The model under review builds one solid part; all positions refer to its coordinate system, in mm. A direction names the side the tool comes from. Coordinates: 2 decimals unless noted, no trailing zeros. Order: outer loops, then holes, each group sorted by start corner. A loop starts at its lowest first (then second) coordinate and runs counter-clockwise, first axis right, second up. Notation, with made-up numbers: M -24,62 L -17,62 A18 ccw -17,81 Z; hole C -6.75,75 d6. An arc over 180 degrees is marked long. One line per item, written item: value.
```python
from build123d import *

# Parameters (mm, degrees)
FILLET1_R          = 0.2
SKETCH2_W          = 1
SKETCH2_H          = 6.101946446
CUT_EXTRUDE1_DEPTH = 1


with BuildPart() as part:
    # Sketch1 → Revolve1 (revolve)
    with BuildSketch(Plane.XY, mode=Mode.PRIVATE) as revolve1_sk:
        Polygon((-6.402554748, 1.5), (-43, 1.5), (-43, 0), (16, 0), (20, 0), (20, 2.75), (18.5, 2.75), (18.5, 1.25), (16, 1.25), (16, 4), (0, 4), (0, 3.603313767), (-1.581765583, 2.560980975), align=None)
    revolve(revolve1_sk.sketch.rotate(Axis((-43, 0, 0), (1, 0, 0)), 90), axis=Axis((-43, 0, 0), (1, 0, 0)))

    # Fillet1
    fillet1_edges = [part.edges().sort_by_distance(p)[0] for p in [
        (0, 0, -4),
        (16, 0, -4),
    ]]
    fillet(fillet1_edges, radius=FILLET1_R)

    # Sketch2 → Cut-Extrude1 (cut)
    with BuildSketch(Plane(origin=(20, 0, 0), x_dir=(0, 0, -1), z_dir=(1, 0, 0))):
        with Locations((0, 0.058366444)):
            Rectangle(SKETCH2_W, SKETCH2_H)
    extrude(amount=-CUT_EXTRUDE1_DEPTH, mode=Mode.SUBTRACT)


solid = part.part
```
(1) Tool access review of faces 4 (the flat face through (16, -1, 1)), 5 (the cylindrical face through (-24.96, -0.45, 1.43)), 6 (the cylindrical face through (19.24, 2.44, 1.27)), 7 (the flat face through (19.5, 0, 0.5)), 8 (the flat face through (20, 0, -1)): name each direction out of +Z, -Z, +X, -X, +Y, -Y from which nothing blocks a thin tool from reaching the whole face with its end or side.
Geometry results:
face 4: none
face 5: -X
face 6: +X
face 7: +X, +Y, -Y
face 8: +Z, -Z, +X, +Y, -Y
(2) Mouldability with a two-part tool opening along X and no side actions: class faces 1 (the flat face through (19.5, 0, -0.5)), 2 (the conical face through (-4.6, -0.6, 1.8)), 3 (the cylindrical face through (17.23, -0.05, -1.25)) as +X half, -X half, draft (parallel to the pull), parting line (faces both ways), or undercut.
Geometry results:
face 1: draft
face 2: -X half
face 3: undercut
(3) We need section A-A, the plane y = 0. State the section outline as (x, z) points, plus the area to 3 significant figures.
Geometry results:
outline: M -43,-1.5 L -6.4,-1.5 L -1.58,-2.56 L 0,-3.6 L 0,-3.8 A0.2 ccw 0.2,-4 L 15.8,-4 A0.2 ccw 16,-3.8 L 16,-1.25 L 18.5,-1.25 L 18.5,-2.75 L 20,-2.75 L 20,-0.5 L 19,-0.5 L 19,0.5 L 20,0.5 L 20,2.75 L 18.5,2.75 L 18.5,1.25 L 16,1.25 L 16,3.8 A0.2 ccw 15.8,4 L 0.2,4 A0.2 ccw 0,3.8 L 0,3.6 L -1.58,2.56 L -6.4,1.5 L -43,1.5 Z
area: 281 mm2
(4) We need section B-B, the plane x = -11.5. State the section outline as (y, z) points, plus the area to 3 significant figures.
Geometry results:
outline: C 0,0 d3
area: 7.07 mm2
(5) For L1, parallel to Y at x = -36.5, z = 0; L2, parallel to X at y = 1, z = 1; L3, parallel to Y at x = -2.5, z = 2, list the stretches that pass through material, from the lowest coordinate up.
Geometry results:
L1: y = -1.5 to 1.5
L2: x = -43 to 16, 18.5 to 20
L3: y = -1.25 to 1.25
(6) Insertion check: pin 1 Ø0.8 at (y, z) = (0.5, 0) entering from +X; pin 2 Ø1.1 at (x, y) = (19.5, 1) entering from -Z; pin 3 Ø0.8 at (x, y) = (19.5, -0.5) entering from +Z. Each pin has a flat end and moves straight along its axis. Give the tip position at first contact, or say it passes through.
Geometry results:
pin 1: stops at x = 19
pin 2: stops at z = -2.71
pin 3: stops at z = 2.75
